Verification items for the finished model (mm, model axes). A direction names the side the tool comes from. Give positions to 0.01 mm unless a question says otherwise; leave off trailing zeros. Write each loop counter-clockwise with the first axis right and the second up, starting at its lowest first coordinate (ties: lowest second). Pieces come first, ordered by that corner, then holes. Notation, with made-up numbers: (80, 36) - (107, 36) arc R19 cw to (107, 68) - close; hole circle Ø4 at (65, -32.75). An arc over 180 degrees is marked (long way). Answer as a JSON object with one key per item and string values. Group by question number.
Item 1: Sectioned sample at B-B, the plane z = 3.9. Record the boundary of the cut face in (x, y).
Item 2: Tool access check on faces 1 (the face through (74, 23, 6)), 2 (the face through (24, 12, 5.5)), 3 (the face through (107, 12, 8)). Record the directions out of +Z, -Z, +X, -X, +Y, -Y that give a thin tool (end or side, any length) a straight path to the whole face; none if there is none.
Item 3: Scan lines: line 1 along Y through (x, z) = (13.5, 8.75); line 2 along Z through (x, y) = (76, 11.5); line 3 along Y through (x, z) = (134, 4.05). Record each from-to range of solid material in increasing order. Write a range as [from, to].
Item 4: Draft check along X on faces 4 (the face through (150, 11, 6)), 5 (the face through (0, 11, 6)), 6 (the face through (74, 12, 3)), 7 (the face through (136.86, 12.4, 4.23)). Enter one of: +X half, -X half, draft (parallel to the pull), parting line (faces both ways), or undercut.
Item 5: Sectioned sample at A-A, the plane x = 52. Record the boundary of the cut face in (y, z).
Item 6: Go/stop test with flat-tipped pins: pin 1 (1.8 mm diameter, centred on x = 16, y = 10.5, fed in from -Z); pin 2 (1.8 mm diameter, centred on x = 110, y = 11, fed in from -Z); pin 3 (5 mm diameter, centred on x = 126, y = 11.5, fed in from +Z). Record where each tip stops, or that it passes through.
Item 7: Sectioned sample at C-C, the plane y = 18. Record the boundary of the cut face in (x, z).
Item 8: Sectioned sample at D-D, the plane x = 126. Record the boundary of the cut face in (y, z), and give its area (3 significant figures).
```python
from build123d import *

# Parameters (mm, degrees)
BOX029_W          = 30
BOX029_H          = 22
BOX029_DEPTH      = 1.5
BOX030_W          = 27
BOX030_H          = 22
BOX030_DEPTH      = 1.5
BOX028_W          = 30
BOX028_H          = 22
BOX028_DEPTH      = 1.5
BOX027_W          = 30
BOX027_H          = 22
BOX027_DEPTH      = 1.5
BOX026_W          = 30
BOX026_H          = 22
BOX026_DEPTH      = 1.5
BOX025_W          = 150
BOX025_H          = 23
BOX025_DEPTH      = 1
CYLINDER006_R     = 3
CYLINDER006_DEPTH = 2.5
CYLINDER005_R     = 3
CYLINDER005_DEPTH = 2.5
CYLINDER007_R     = 3
CYLINDER007_DEPTH = 2.5
CYLINDER004_R     = 3
CYLINDER004_DEPTH = 2.5
BOX001_W          = 150
BOX001_H          = 23
BOX001_DEPTH      = 5


with BuildPart() as cube007:
    # Box029 → Box029 (new body)
    with BuildSketch(Plane(origin=(92, 0.5, 8), x_dir=(1, 0, 0), z_dir=(0, 0, 1))):
        with Locations((15, 11)):
            Rectangle(BOX029_W, BOX029_H)
    extrude(amount=BOX029_DEPTH)


with BuildPart() as cube008:
    # Box030 → Box030 (new body)
    with BuildSketch(Plane(origin=(122.5, 0.5, 8), x_dir=(1, 0, 0), z_dir=(0, 0, 1))):
        with Locations((13.5, 11)):
            Rectangle(BOX030_W, BOX030_H)
    extrude(amount=BOX030_DEPTH)


with BuildPart() as cube006:
    # Box028 → Box028 (new body)
    with BuildSketch(Plane(origin=(61.5, 0.5, 8), x_dir=(1, 0, 0), z_dir=(0, 0, 1))):
        with Locations((15, 11)):
            Rectangle(BOX028_W, BOX028_H)
    extrude(amount=BOX028_DEPTH)


with BuildPart() as cube005:
    # Box027 → Box027 (new body)
    with BuildSketch(Plane(origin=(31, 0.5, 8), x_dir=(1, 0, 0), z_dir=(0, 0, 1))):
        with Locations((15, 11)):
            Rectangle(BOX027_W, BOX027_H)
    extrude(amount=BOX027_DEPTH)


with BuildPart() as remove_holes:
    # Box026 → Box026 (new body)
    with BuildSketch(Plane(origin=(0.5, 0.5, 8), x_dir=(1, 0, 0), z_dir=(0, 0, 1))):
        with Locations((15, 11)):
            Rectangle(BOX026_W, BOX026_H)
    extrude(amount=BOX026_DEPTH)

    # Fusion027: union Cube007, Cube008, Cube006, Cube005
    add(cube007.part)
    add(cube008.part)
    add(cube006.part)
    add(cube005.part)


with BuildPart() as f_5x_loose:
    # Box025 → Box025 (new body)
    with BuildSketch(Plane.XY.offset(8)):
        with Locations((75, 11.5)):
            Rectangle(BOX025_W, BOX025_H)
    extrude(amount=BOX025_DEPTH)

    # Cut010: cut remove_holes
    add(remove_holes.part, mode=Mode.SUBTRACT)


with BuildPart() as cone002:
    # Cone002 → Cone002 (revolve)
    with BuildSketch(Plane(origin=(40, 11.5, 3), x_dir=(1, 0, 0), z_dir=(0, -1, 0))):
        Polygon((0, 0), (5.1, 0), (1.1, 4.1), (0, 4.1), align=None)
    revolve(axis=Axis((40, 11.5, 3), (0, 0, 1)))


with BuildPart() as cone003:
    # Cone003 → Cone003 (revolve)
    with BuildSketch(Plane(origin=(110, 11.5, 3), x_dir=(1, 0, 0), z_dir=(0, -1, 0))):
        Polygon((0, 0), (5.1, 0), (1.1, 4.1), (0, 4.1), align=None)
    revolve(axis=Axis((110, 11.5, 3), (0, 0, 1)))


with BuildPart() as cylinder006:
    # Cylinder006 → Cylinder006 (new body)
    with BuildSketch(Plane(origin=(24, 11.5, 3), x_dir=(1, 0, 0), z_dir=(0, 0, 1))):
        Circle(CYLINDER006_R)
    extrude(amount=CYLINDER006_DEPTH)


with BuildPart() as cylinder005:
    # Cylinder005 → Cylinder005 (new body)
    with BuildSketch(Plane(origin=(126, 11.5, 3), x_dir=(1, 0, 0), z_dir=(0, 0, 1))):
        Circle(CYLINDER005_R)
    extrude(amount=CYLINDER005_DEPTH)


with BuildPart() as cylinder007:
    # Cylinder007 → Cylinder007 (new body)
    with BuildSketch(Plane(origin=(134, 11.5, 3), x_dir=(1, 0, 0), z_dir=(0, 0, 1))):
        Circle(CYLINDER007_R)
    extrude(amount=CYLINDER007_DEPTH)


with BuildPart() as removals:
    # Cylinder004 → Cylinder004 (new body)
    with BuildSketch(Plane(origin=(16, 11.5, 3), x_dir=(1, 0, 0), z_dir=(0, 0, 1))):
        Circle(CYLINDER004_R)
    extrude(amount=CYLINDER004_DEPTH)

    # Fusion002: union Cone002, Cone003, Cylinder006, Cylinder005, Cylinder007
    add(cone002.part)
    add(cone003.part)
    add(cylinder006.part)
    add(cylinder005.part)
    add(cylinder007.part)


with BuildPart() as top_5x_loose:
    # Box001 → Box001 (new body)
    with BuildSketch(Plane.XY.offset(3)):
        with Locations((75, 11.5)):
            Rectangle(BOX001_W, BOX001_H)
    extrude(amount=BOX001_DEPTH)

    # Cut009: cut removals
    add(removals.part, mode=Mode.SUBTRACT)

    # Fusion028: union 5x_loose
    add(f_5x_loose.part)


solid = top_5x_loose.part
```
Geometry check:
{
 "1": {"outline": "(0, 0) - (150, 0) - (150, 23) - (0, 23) - close; hole circle Ø6 at (16, 11.5); hole circle Ø6 at (24, 11.5); hole circle Ø8.44 at (40, 11.5); hole circle Ø8.44 at (110, 11.5); hole circle Ø6 at (126, 11.5); hole circle Ø6 at (134, 11.5)"},
 "2": {"face 1": "+Z, -Z, +X, -X, +Y", "face 2": "-Z", "face 3": "+Z"},
 "3": {"line 1": "[0, 0.5], [22.5, 23]", "line 2": "[3, 8]", "line 3": "[0, 8.5], [14.5, 23]"},
 "4": {"face 4": "+X half", "face 5": "-X half", "face 6": "draft", "face 7": "undercut"},
 "5": {"outline": "(0, 3) - (23, 3) - (23, 9) - (22.5, 9) - (22.5, 8) - (0.5, 8) - (0.5, 9) - (0, 9) - close"},
 "6": {"pin 1": "z = 5.5", "pin 2": "z = 6.79", "pin 3": "z = 8"},
 "7": {"outline": "(0, 3) - (150, 3) - (150, 9) - (149.5, 9) - (149.5, 8) - (122.5, 8) - (122.5, 9) - (122, 9) - (122, 8) - (92, 8) - (92, 9) - (91.5, 9) - (91.5, 8) - (61.5, 8) - (61.5, 9) - (61, 9) - (61, 8) - (31, 8) - (31, 9) - (30.5, 9) - (30.5, 8) - (0.5, 8) - (0.5, 9) - (0, 9) - close"},
 "8": {"outline": "(0, 3) - (8.5, 3) - (8.5, 5.5) - (14.5, 5.5) - (14.5, 3) - (23, 3) - (23, 9) - (22.5, 9) - (22.5, 8) - (0.5, 8) - (0.5, 9) - (0, 9) - close", "area": "101 mm^2"}
}
